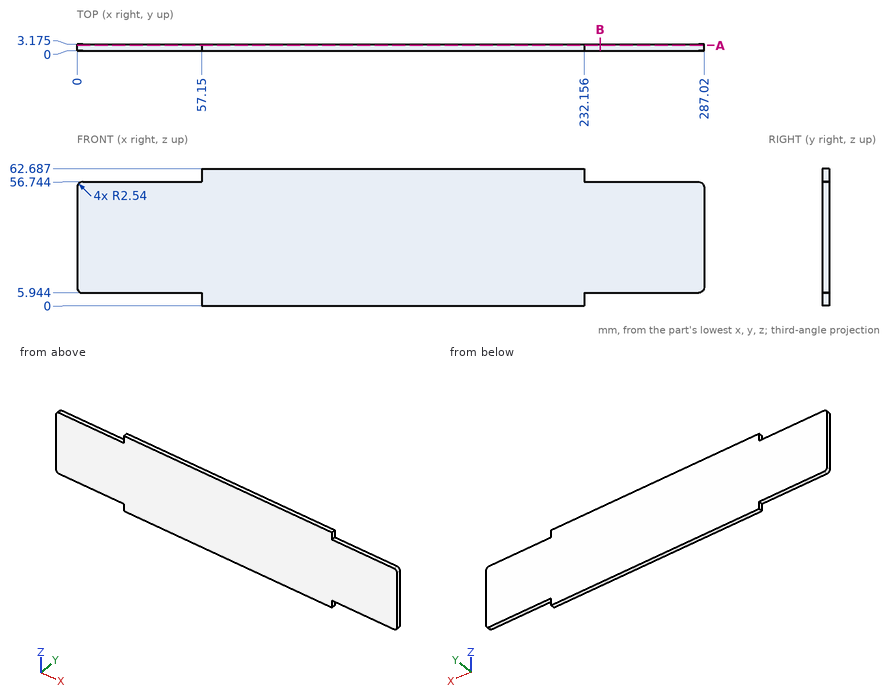
The drawing under review shows one solid part. Ordinate dimensions are in mm from its lowest x, y, z. Round coordinates to 2 decimals unless told otherwise and drop trailing zeros. Order: outer loops, then holes, each group sorted by start corner. A loop starts at its lowest first (then second) coordinate and runs counter-clockwise, first axis right, second up. Notation, with made-up numbers: (78, 49) -> (111, 49) arc R22 ccw to (111, 55) -> close; hole circle Ø9 at (-9, 66). An arc over 180 degrees is marked (long way). Return JSON: item names as keys, results as strings.
1. Take a section at A-A (y = 2.6). Write out the cut boundary in (x, z).
Answer block:
{"outline": "(0, 8.48) arc R2.54 ccw to (2.54, 5.94) -> (57.15, 5.94) -> (57.15, 0) -> (232.16, 0) -> (232.16, 5.94) -> (284.48, 5.94) arc R2.54 ccw to (287.02, 8.48) -> (287.02, 54.2) arc R2.54 ccw to (284.48, 56.74) -> (232.16, 56.74) -> (232.16, 62.69) -> (57.15, 62.69) -> (57.15, 56.74) -> (2.54, 56.74) arc R2.54 ccw to (0, 54.2) -> close"}
2. Insertion check: P1, Ø1, axis at x = 34, y = 1, coming from the -Z side; P2, Ø1, axis at y = 1.5, z = 59.5, coming from the +X side; P3, Ø1, axis at y = 1.5, z = 58.5, coming from the -X side. Each pin has a flat end and moves straight along its axis. Give the tip position at first contact, or say it passes through.
Answer block:
{"P1": "stops at z = 5.94", "P2": "stops at x = 232.16", "P3": "stops at x = 57.15"}
3. For L1, parallel to Z at x = 253.5, y = 2.75; L2, parallel to X at y = 1.05, z = 4.5; L3, parallel to X at y = 1, z = 56 (1 decimal), list the stretches that pass through material, from the lowest coordinate up. Write a range as [from, to].
Answer block:
{"L1": "z = [5.94, 56.74]", "L2": "x = [57.15, 232.16]", "L3": "x = [0.7, 286.3]"}
4. Take a section at B-B (x = 239.5). Write out the cut boundary in (y, z) (1 decimal), then the cut area to 3 significant figures.
Answer block:
{"outline": "(0, 5.9) -> (3.2, 5.9) -> (3.2, 56.7) -> (0, 56.7) -> close", "area": "161 mm²"}
